from build123d import *

# Parameters (mm, degrees)
SKETCH4_W           = 20
SKETCH4_H           = 120
BOSS_EXTRUDE4_DEPTH = 10
SKETCH5_R           = 2.1
CUT_EXTRUDE1_DEPTH  = 10
SKETCH8_W           = 20
SKETCH8_H           = 55
BOSS_EXTRUDE6_DEPTH = 55
SKETCH9_W           = 40.5
SKETCH9_H           = 20.5
CUT_EXTRUDE2_DEPTH  = 20
SKETCH11_R          = 2.6
CUT_EXTRUDE3_DEPTH  = 50
SKETCH12_W          = 10
SKETCH12_H          = 55
BOSS_EXTRUDE7_DEPTH = 50
SKETCH15_R          = 12.5
CUT_EXTRUDE4_DEPTH  = 10
SKETCH17_W          = 50
SKETCH17_H          = 12.25
CUT_EXTRUDE6_DEPTH  = 10
CHAMFER1_SIZE       = 12.5
FILLET1_R           = 2
CHAMFER2_SIZE       = 5


with BuildPart() as part:
    # Sketch4 → Boss-Extrude4 (new body)
    with BuildSketch(Plane(origin=(0, 0, 0), x_dir=(1, 0, 0), z_dir=(0, 1, 0))):
        with Locations((10, 60)):
            Rectangle(SKETCH4_W, SKETCH4_H)
    extrude(amount=BOSS_EXTRUDE4_DEPTH)

    # Sketch5 → Cut-Extrude1 (cut)
    with BuildSketch(Plane(origin=(0, 10, 0), x_dir=(1, 0, 0), z_dir=(0, 1, 0))):
        with Locations(Location((10, 105, 0), (0, 0, 270))):
            Circle(SKETCH5_R)
        with Locations(Location((10, 15, 0), (0, 0, 270))):
            Circle(SKETCH5_R)
    extrude(amount=-CUT_EXTRUDE1_DEPTH, mode=Mode.SUBTRACT)

    # Sketch8 → Boss-Extrude6 (add)
    with BuildSketch(Plane(origin=(0, 10, 0), x_dir=(1, 0, 0), z_dir=(0, 1, 0))):
        with Locations((10, 52.5)):
            Rectangle(SKETCH8_W, SKETCH8_H)
    extrude(amount=BOSS_EXTRUDE6_DEPTH)

    # Sketch9 → Cut-Extrude2 (cut)
    with BuildSketch(Plane.ZY):
        with Locations((-49.75, 44.75)):
            Rectangle(SKETCH9_W, SKETCH9_H)
    extrude(amount=-CUT_EXTRUDE2_DEPTH, mode=Mode.SUBTRACT)

    # Sketch11 → Cut-Extrude3 (cut, symmetric)
    with BuildSketch(Plane.XY.offset(-70)):
        with Locations((10, 44.75)):
            Circle(SKETCH11_R)
    extrude(amount=CUT_EXTRUDE3_DEPTH, both=True, mode=Mode.SUBTRACT)

    # Sketch12 → Boss-Extrude7 (add)
    with BuildSketch(Plane.ZY):
        with Locations((-75, 37.5)):
            Rectangle(SKETCH12_W, SKETCH12_H)
    extrude(amount=BOSS_EXTRUDE7_DEPTH)

    # Sketch15 → Cut-Extrude4 (cut)
    with BuildSketch(Plane.XY.offset(-70)):
        with Locations((-24.72528445, 45.000219356)):
            Circle(SKETCH15_R)
        with BuildLine():
            ThreePointArc((-7.62528445, 60.500219356), (-9.22528445, 62.100219356), (-10.82528445, 60.500219356))
            Line((-10.82528445, 60.500219356), (-9.22528445, 60.500219356))
            Line((-9.22528445, 60.500219356), (-9.22528445, 58.900219356))
            ThreePointArc((-9.22528445, 58.900219356), (-8.0939136, 59.368848506), (-7.62528445, 60.500219356))
        make_face()
        with BuildLine():
            Line((-9.22528445, 60.500219356), (-10.82528445, 60.500219356))
            ThreePointArc((-10.82528445, 60.500219356), (-10.3566553, 59.368848506), (-9.22528445, 58.900219356))
            Line((-9.22528445, 58.900219356), (-9.22528445, 60.500219356))
        make_face()
        with BuildLine():
            ThreePointArc((-7.62528445, 29.500219356), (-8.0939136, 30.631590206), (-9.22528445, 31.100219356))
            Line((-9.22528445, 31.100219356), (-9.22528445, 29.500219356))
            Line((-9.22528445, 29.500219356), (-10.82528445, 29.500219356))
            ThreePointArc((-10.82528445, 29.500219356), (-9.22528445, 27.900219356), (-7.62528445, 29.500219356))
        make_face()
        with BuildLine():
            Line((-9.22528445, 29.500219356), (-9.22528445, 31.100219356))
            ThreePointArc((-9.22528445, 31.100219356), (-10.3566553, 30.631590206), (-10.82528445, 29.500219356))
            Line((-10.82528445, 29.500219356), (-9.22528445, 29.500219356))
        make_face()
        with BuildLine():
            ThreePointArc((-38.62528445, 29.500219356), (-39.0939136, 30.631590206), (-40.22528445, 31.100219356))
            Line((-40.22528445, 31.100219356), (-40.22528445, 29.500219356))
            Line((-40.22528445, 29.500219356), (-38.62528445, 29.500219356))
        make_face()
        with BuildLine():
            Line((-40.22528445, 29.500219356), (-40.22528445, 31.100219356))
            ThreePointArc((-40.22528445, 31.100219356), (-41.3566553, 28.368848506), (-38.62528445, 29.500219356))
            Line((-38.62528445, 29.500219356), (-40.22528445, 29.500219356))
        make_face()
        with BuildLine():
            Line((-40.22528445, 58.900219356), (-40.22528445, 60.500219356))
            Line((-40.22528445, 60.500219356), (-38.62528445, 60.500219356))
            ThreePointArc((-38.62528445, 60.500219356), (-41.3566553, 61.631590206), (-40.22528445, 58.900219356))
        make_face()
        with BuildLine():
            Line((-38.62528445, 60.500219356), (-40.22528445, 60.500219356))
            Line((-40.22528445, 60.500219356), (-40.22528445, 58.900219356))
            ThreePointArc((-40.22528445, 58.900219356), (-39.0939136, 59.368848506), (-38.62528445, 60.500219356))
        make_face()
    extrude(amount=-CUT_EXTRUDE4_DEPTH, mode=Mode.SUBTRACT)

    # Sketch17 → Cut-Extrude6 (cut)
    with BuildSketch(Plane.XY.offset(-70)):
        with Locations((-25, 16.125)):
            Rectangle(SKETCH17_W, SKETCH17_H)
    extrude(amount=-CUT_EXTRUDE6_DEPTH, mode=Mode.SUBTRACT)

    # Chamfer1
    chamfer1_edges = [part.edges().sort_by_distance(p)[0] for p in [
        (0, 22.25, -75),
    ]]
    chamfer(chamfer1_edges, length=CHAMFER1_SIZE)

    # Fillet1
    fillet1_edges = [part.edges().sort_by_distance(p)[0] for p in [
        (-50, 22.25, -75),
        (0, 4.875, -120),
        (10, 65, -25),
        (-50, 65, -75),
        (20, 5, -120),
    ]]
    fillet(fillet1_edges, radius=FILLET1_R)

    # Chamfer2
    chamfer2_edges = [part.edges().sort_by_distance(p)[0] for p in [
        (0, 22.125, -70),
        (0, 60, -70),
    ]]
    chamfer(chamfer2_edges, length=CHAMFER2_SIZE)


solid = part.part
Check sheet for the modelled part. Datum: model origin and axes. Units: mm. A direction names the side the tool comes from. Round coordinates to 2 decimals unless told otherwise and drop trailing zeros. Loops run counter-clockwise (first coordinate to the right, second up) from the corner with the lowest first, then second, coordinate; pieces in that order, holes last.
1. Sectioned sample at A-A on z = -35.5. Record the boundary of the cut face in (x, y), and give its area (3 significant figures).
2. Gauge pin test, flat ends, axial feed: pin 1 Ø4 at (x, z) = (10, -15) entering from +Y; pin 2 Ø1.5 at (x, y) = (-6, 18.5) entering from +Z; pin 3 Ø10 at (x, z) = (6.5, -105.5) entering from +Y; pin 4 Ø16.5 at (x, y) = (-18, 44.5) entering from -Z. Record the tip position at first contact, or that the pin passes through.
3. Set-up check for faces 5 (the flat face through (10, 34.5, -50)), 6 (the flat face through (-14.5, 37.1, -80)), 7 (the flat face through (9.9, 10, -12.7)): record each of +Z, -Z, +X, -X, +Y, -Y from which the full face is reachable in a straight line by a thin tool's end or side.
4. Sectioned sample at C-C on x = -21.5. Record the boundary of the cut face in (y, z), and give its area (3 significant figures).
5. Mould release check, pull along Z, two halves, no side actions. Record for faces 1 (the cylindrical face through (10.09, 5.07, -107.1)), 2 (the flat face through (-50, 44, -75)), 3 (the flat face through (-15, 34, -70)), 4 (the flat face through (9, 5, -120)): released by +Z, released by -Z, zero draft, split by the parting line, or undercut.
6. Sectioned sample at D-D on z = -105. Record the boundary of the cut face in (x, y), and give its area (3 significant figures).
7. Sectioned sample at B-B on x = 4. Record the boundary of the cut face in (y, z).
8. Scan lines: probe 1 along Y at (x, z) = (10, -74.25); probe 2 along Y at (x, z) = (12.5, -50.5); probe 3 along X at (y, z) = (2, -105). Record each from-to range of solid material in increasing order.
Recorded:
1. outline: (0, 0) - (20, 0) - (20, 34.5) - (0, 34.5) - close; (0, 55) - (20, 55) - (20, 65) - (0, 65) - close
1. area: 890 mm2
2. pin 1: passes through
2. pin 2: stops at z = -70
2. pin 3: stops at y = 10
2. pin 4: stops at z = -80
3. face 5: +X, -X
3. face 6: -Z, +X, -X, +Y
3. face 7: +Z, +X, -X, +Y
4. outline: (22.25, -80) - (32.92, -80) - (32.92, -70) - (22.25, -70) - close; (57.08, -80) - (65, -80) - (65, -70) - (57.08, -70) - close
4. area: 186 mm2
5. face 1: undercut
5. face 2: zero draft
5. face 3: undercut
5. face 4: released by -Z
6. outline: (-0.25, 10) - (0, 9.75) - (0, 0) - (7.9, 0) - (7.9, 10) - close; (12.1, 0) - (20, 0) - (20, 10) - (12.1, 10) - close
6. area: 158 mm2
7. outline: (0, -120) - (10, -120) - (10, -80) - (65, -80) - (65, -27) arc R2 ccw to (63, -25) - (10, -25) - (10, 0) - (0, 0) - close; hole (34.5, -70) - (55, -70) - (55, -29.5) - (34.5, -29.5) - close
8. probe 1: y = 0 to 42.15, 47.35 to 65
8. probe 2: y = 0 to 34.5, 55 to 65
8. probe 3: x = 0 to 7.9, 12.1 to 20
